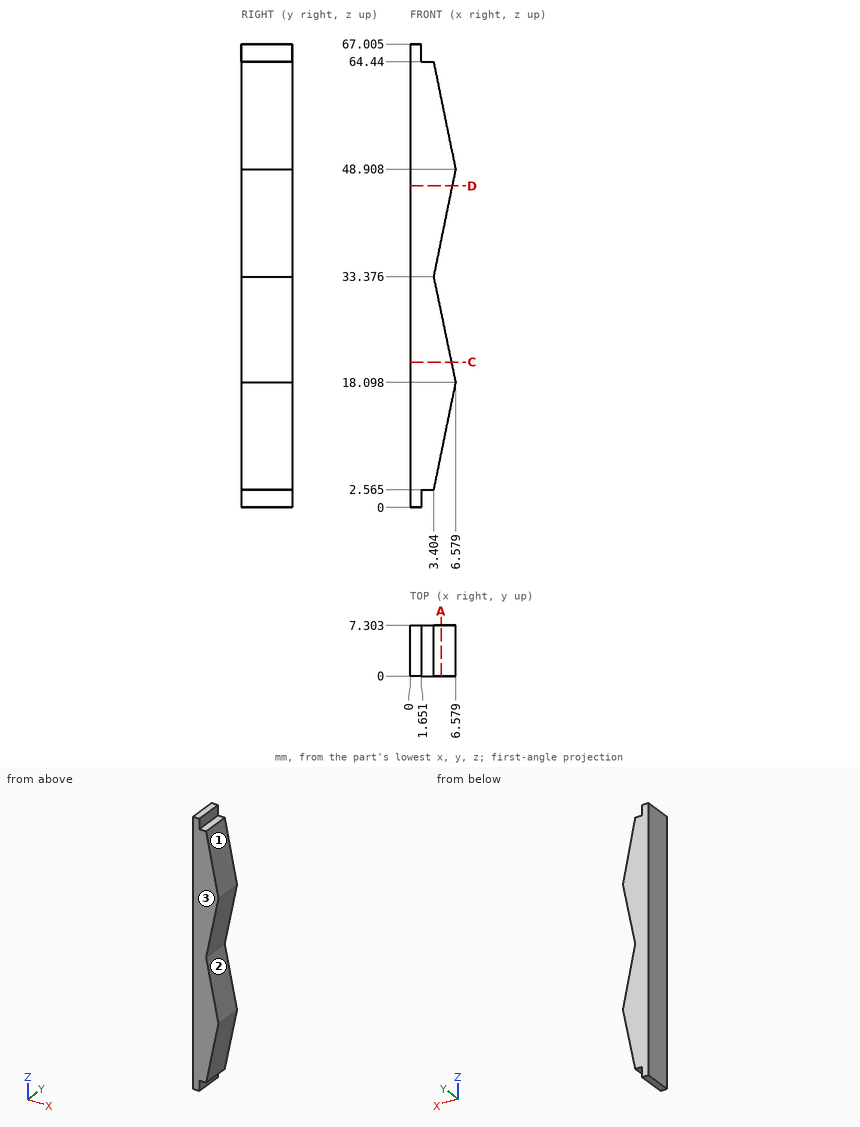
Input: dimensioned drawing with shaded views. Units: mm. Origin: part minimum x, y, z. Round coordinates to 2 decimals unless told otherwise and drop trailing zeros. Order: outer loops, then holes, each group sorted by start corner. A loop starts at its lowest first (then second) coordinate and runs counter-clockwise, first axis right, second up. Notation, with made-up numbers: (62.5, 13) - (116.5, 13) arc R12 cw to (116.5, 33) - close; hole circle Ø6 at (55.5, 1.5). An arc over 180 degrees is marked (long way). Answer as a JSON object with one key per item and string values. Group by question number.
(1) Cut plane A-A (x = 4.5). Return loops of the section in (y, z), then the cut area to 3 significant figures.
(2) Cut plane C-C (z = 21). Return loops of the section in (x, y) (1 decimal).
(3) Material intervals for probe 1 along Z at (x, y) = (2, 6.5) (1 decimal); probe 2 along X at (y, z) = (5, 36); probe 3 along X at (y, z) = (1.5, 13.5), sorted ascending. Write a range as from..to.
(4) Cut plane D-D (z = 46.5). Return loops of the section in (x, y).
(5) Draft query along Z for the marked faces 1, 2 and 3. Return one class per face: released by +Z, released by -Z, zero draft, split by the parting line, or undercut.
(6) Pin query (flat end, axial travel): P1, Ø1.4, axis at x = 2.5, y = 2, coming from the +Z side; P2, Ø1.9, axis at x = 2.5, y = 3.5, coming from the -Z side; P3, Ø3, axis at y = 2, z = 1.5, coming from the +X side; P4, Ø2, axis at y = 6, z = 29, coming from the +X side. Return the tip coordinate at first contact, or that it passes through.
Here are the results:
{
 "1": {"outline": "(0, 7.93) - (7.3, 7.93) - (7.3, 28.1) - (0, 28.1) - close; (0, 38.74) - (7.3, 38.74) - (7.3, 59.08) - (0, 59.08) - close", "area": "296 mm^2"},
 "2": {"outline": "(0, 0) - (6, 0) - (6, 7.3) - (0, 7.3) - close"},
 "3": {"probe 1": "z = 2.6..64.4", "probe 2": "x = 0..3.94", "probe 3": "x = 0..5.64"},
 "4": {"outline": "(0, 0) - (6.09, 0) - (6.09, 7.3) - (0, 7.3) - close"},
 "5": {"face 1": "released by +Z", "face 2": "undercut", "face 3": "zero draft"},
 "6": {"P1": "stops at z = 64.44", "P2": "stops at z = 0", "P3": "stops at x = 3.49", "P4": "stops at x = 4.52"}
}
